from build123d import *

# Parameters (mm, degrees)
ESQUISSE1_R               = 4
BOSS_EXTRU_1_DEPTH        = 90
ESQUISSE2_R               = 1.25
ENL_V_MAT_EXTRU_1_DEPTH   = 10
TROU_TARAUD_M3X0_51_D     = 2.5
TROU_TARAUD_M3X0_51_DEPTH = 12.5
TROU_TARAUD_M3X0_51_TIP   = 0.751075774
ESQUISSE6_R               = 3
ENL_V_MAT_EXTRU_2_DEPTH   = 91.177602649


with BuildPart() as part:
    # Esquisse1 → Boss.-Extru.1 (new body)
    with BuildSketch(Plane.XY):
        Circle(ESQUISSE1_R)
    extrude(amount=-BOSS_EXTRU_1_DEPTH)

    # Esquisse2 → Enlèv. mat.-Extru.1 (cut, symmetric)
    with BuildSketch(Plane(origin=(0, 0, 0), x_dir=(1, 0, 0), z_dir=(0, 1, 0))):
        with Locations(Location((0, 16.5, 0), (0, 0, 270))):
            Circle(ESQUISSE2_R)
    extrude(amount=ENL_V_MAT_EXTRU_1_DEPTH, both=True, mode=Mode.SUBTRACT)

    # Trou taraudé M3x0.51
    with Locations(Plane(origin=(0, 0, -90), x_dir=(-1, 0, 0), z_dir=(0, 0, -1))):
        with Locations((0, 0)):
            Hole(TROU_TARAUD_M3X0_51_D / 2, depth=TROU_TARAUD_M3X0_51_DEPTH)
            with Locations((0, 0, -(TROU_TARAUD_M3X0_51_DEPTH + TROU_TARAUD_M3X0_51_TIP / 2))):  # 118° drill point
                Cone(0, TROU_TARAUD_M3X0_51_D / 2, TROU_TARAUD_M3X0_51_TIP, mode=Mode.SUBTRACT)

    # Esquisse6 → Enlèv. mat.-Extru.2 (cut, through all)
    with BuildSketch(Plane.XY):
        Circle(ESQUISSE6_R)
    extrude(amount=-ENL_V_MAT_EXTRU_2_DEPTH, mode=Mode.SUBTRACT)


solid = part.part
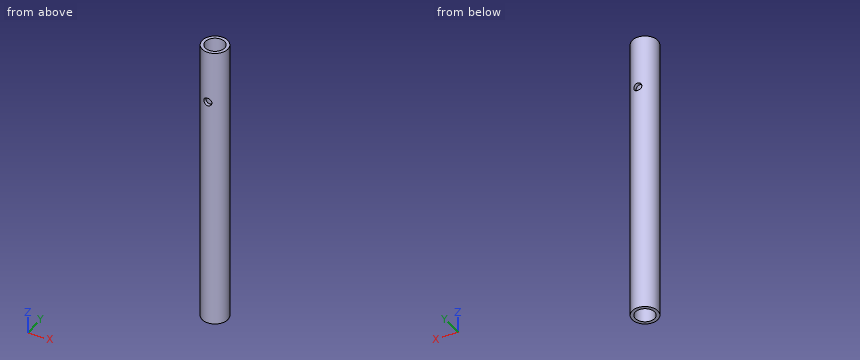
Source: CAD feature listing. Evaluate the final solid. Frame: model axes, mm. Round coordinates to 2 decimals unless told otherwise and drop trailing zeros. Loops run counter-clockwise (first coordinate to the right, second up) from the corner with the lowest first, then second, coordinate; pieces in that order, holes last.
Q1. First-contact query: P1, Ø4, axis at y = 1.5, z = -61.5, coming from the -X side; P2, Ø2, axis at x = 0, z = -16.5, coming from the +Y side. Flat tips, straight axial feed; report the tip coordinate or a pass-through.
Q2. Section B-B, the plane z = -16.5. Return loops of the section in (x, y), plus the area to 3 significant figures.
Q3. Ray query, line 1 (Z direction, x = 0, y = -3.5); line 2 (Y direction, x = -2.75, z = -61.5); line 3 (X direction, y = 3.25, z = -16.5). Return the intervals inside material, ascending.
Q4. Section A-A, the plane y = 0. Return loops of the section in (x, z), plus the area to 3 significant figures.
Solutions:
1. P1: stops at x = -4
1. P2: passes through
2. outline: (-1.25, -3.8) - (-1.25, -2.73) arc R3 cw to (-1.25, 2.73) - (-1.25, 3.8) arc R4 ccw to start; (1.25, -3.8) arc R4 ccw to (1.25, 3.8) - (1.25, 2.73) arc R3 cw to (1.25, -2.73) - close
2. area: 16.9 mm2
3. line 1: z = -90 to -17.75, -15.25 to 0
3. line 2: y = -2.9 to -1.2, 1.2 to 2.9
3. line 3: x = -2.33 to -1.25, 1.25 to 2.33
4. outline: (-4, -90) - (-3, -90) - (-3, 0) - (-4, 0) - close; (3, -90) - (4, -90) - (4, 0) - (3, 0) - close
4. area: 180 mm2
